Work out the finished part from the listing and answer in its coordinate system (mm). A direction names the side the tool comes from. Give positions to 0.01 mm unless a question says otherwise; leave off trailing zeros. Write each loop counter-clockwise with the first axis right and the second up, starting at its lowest first coordinate (ties: lowest second). Pieces come first, ordered by that corner, then holes.
1) Determine the mould class of faces 6 (the face through (-107, 7, 2)), 7 (the face through (9.493, 0.986, -0.36)), 8 (the face through (-2.44, 0.99, -0.54)) for opening direction X: pulls with the +X half, pulls with the -X half, needs draft (parallel to the pull), parting line crosses it, or undercut.
2) A tool of negligible diameter and unlimited length cuts with its end or side. For faces 1 (the face through (9.493, 13.986, -0.36)), 2 (the face through (-90, 15, 1)), 3 (the face through (-12.3, 4.9, -2)), 4 (the face through (-10.633, 3.595, -0.479)), 5 (the face through (-4.88, 13.99, -1.08)), from which of +Z, -Z, +X, -X, +Y, -Y can it reach the whole face along a straight path? Write none if from no direction.
3) Find section A-A (z = -6.75). Determine the outline of the cut face in (x, y), plus the area to 3 significant figures.
4) Find section B-B (x = -11.5). Determine the outline of the cut face in (y, z).
5) Find section C-C (x = -186). Determine the outline of the cut face in (y, z).
6) Given pin 1 Ø2.5 at (x, y) = (-13, 6.5) entering from -Z; pin 2 Ø5.5 at (x, y) = (-70, 9) entering from -Z; pin 3 Ø5 at (x, y) = (-191.5, 7.5) entering from +Z, each flat-ended and moving along its own axis, determine where each tip first touches the part or whether it passes through.
7) Straight lines are drawn through the part: probe 1 along Y at (x, z) = (-11.5, 2.6); probe 2 along Y at (x, z) = (-145, 1.25); probe 3 along Z at (x, y) = (-192, 0.85). For each, find the intervals that lie inside material, in ascending order.
```python
from build123d import *

# Parameters (mm, degrees)
SKETCH1_R                         = 2.5
BOSS_EXTRUDE3_DEPTH               = 2
SKETCH5_W                         = 2
SKETCH5_H                         = 11
BOSS_EXTRUDE4_DEPTH               = 197.88316
SKETCH6_R                         = 5
BOSS_EXTRUDE5_DEPTH               = 2
SKETCH8_W                         = 2
SKETCH8_H                         = 11
BOSS_EXTRUDE6_DEPTH               = 4
CUT_EXTRUDE8_REACH                = 209.363
SKETCH10_R                        = 2
SKETCH10_R_2                      = 1.5
SKETCH11_R                        = 4
SKETCH11_R_2                      = 2.5
BOSS_EXTRUDE7_DEPTH               = 4
CUT_EXTRUDE9_REACH                = 209.363
SKETCH12_R                        = 2.5
M3_5X0_6_TAPPED_HOLE2_D           = 2.9
M3_5X0_6_TAPPED_HOLE2_DEPTH       = 2
M3_5X0_6_TAPPED_HOLE2_CSINK_D     = 3.55
M3_5X0_6_TAPPED_HOLE2_CSINK_ANGLE = 90
M3_5X0_6_TAPPED_HOLE2_TIP         = 0.871247898
FILLET1_R                         = 1


with BuildPart() as part:
    # Sketch1 → Boss-Extrude3 (new body)
    with BuildSketch(Plane(origin=(0, 0, 0), x_dir=(1, 0, 0), z_dir=(0, 1, 0))):
        with BuildLine():
            Line((-206.5, 4), (-8.61684397, 4))
            ThreePointArc((-8.61684397, 4), (9.5, 0), (-8.61684397, -4))
            Line((-8.61684397, -4), (-206.5, -4))
            Line((-206.5, -4), (-206.5, 4))
        make_face()
        with Locations(Location((0, 0, 0), (0, 0, 270))):
            Circle(SKETCH1_R, mode=Mode.SUBTRACT)
    extrude(amount=BOSS_EXTRUDE3_DEPTH)

    # Sketch5 → Boss-Extrude4 (add)
    with BuildSketch(Plane.ZY.offset(206.5)):
        with Locations((3, 7.5)):
            Rectangle(SKETCH5_W, SKETCH5_H)
    extrude(amount=-BOSS_EXTRUDE4_DEPTH)


with BuildPart() as boss_extrude5_tool:
    # Sketch6 → Boss-Extrude5 (new body)
    with BuildSketch(Plane(origin=(0, 13, 0), x_dir=(1, 0, 0), z_dir=(0, 1, 0))):
        with BuildLine():
            Line((-206.5, 4), (-8.61684397, 4))
            ThreePointArc((-8.61684397, 4), (9.5, 0), (-8.61684397, -4))
            Line((-8.61684397, -4), (-206.5, -4))
            Line((-206.5, -4), (-206.5, 4))
        make_face()
        with Locations(Location((0, 0, 0), (0, 0, 270))):
            Circle(SKETCH6_R, mode=Mode.SUBTRACT)
    extrude(amount=BOSS_EXTRUDE5_DEPTH)


with BuildPart() as part_1:
    add(part.part)


with BuildPart() as part_2:
    # Boss-Extrude5: joined with boss_extrude5_tool
    add(part_1.part.fuse(boss_extrude5_tool.part, tol=0.00001))

    # Sketch8 → Boss-Extrude6 (add)
    with BuildSketch(Plane(origin=(-8.61684397, 0, 0), x_dir=(0, 0, -1), z_dir=(1, 0, 0))):
        with Locations((-3, 7.5)):
            Rectangle(SKETCH8_W, SKETCH8_H)
    extrude(amount=BOSS_EXTRUDE6_DEPTH)

    # Sketch10 → Cut-Extrude8 (cut, up to next)
    with BuildSketch(Plane(origin=(0, 0, 2), x_dir=(-1, 0, 0), z_dir=(0, 0, -1)), mode=Mode.PRIVATE) as cut_extrude8_sk1:
        with Locations((201.5, 7.5)):
            Circle(SKETCH10_R)
    cut_extrude8_tool1 = extrude(cut_extrude8_sk1.sketch, amount=-CUT_EXTRUDE8_REACH, mode=Mode.PRIVATE) & part_2.part
    # Sketch10 → Cut-Extrude8 (cut, up to next)
    with BuildSketch(Plane(origin=(0, 0, 2), x_dir=(-1, 0, 0), z_dir=(0, 0, -1)), mode=Mode.PRIVATE) as cut_extrude8_sk2:
        with Locations((191.5, 7.5)):
            Circle(SKETCH10_R)
    cut_extrude8_tool2 = extrude(cut_extrude8_sk2.sketch, amount=-CUT_EXTRUDE8_REACH, mode=Mode.PRIVATE) & part_2.part
    # Sketch10 → Cut-Extrude8 (cut, up to next)
    with BuildSketch(Plane(origin=(0, 0, 2), x_dir=(-1, 0, 0), z_dir=(0, 0, -1)), mode=Mode.PRIVATE) as cut_extrude8_sk3:
        with Locations((158.9, 7)):
            Circle(SKETCH10_R_2)
    cut_extrude8_tool3 = extrude(cut_extrude8_sk3.sketch, amount=-CUT_EXTRUDE8_REACH, mode=Mode.PRIVATE) & part_2.part
    # Sketch10 → Cut-Extrude8 (cut, up to next)
    with BuildSketch(Plane(origin=(0, 0, 2), x_dir=(-1, 0, 0), z_dir=(0, 0, -1)), mode=Mode.PRIVATE) as cut_extrude8_sk4:
        with Locations((140.9, 7)):
            Circle(SKETCH10_R_2)
    cut_extrude8_tool4 = extrude(cut_extrude8_sk4.sketch, amount=-CUT_EXTRUDE8_REACH, mode=Mode.PRIVATE) & part_2.part
    add(cut_extrude8_tool1.solids().sort_by_distance((-201.5, 7.5, 2))[0], mode=Mode.SUBTRACT)
    add(cut_extrude8_tool2.solids().sort_by_distance((-191.5, 7.5, 2))[0], mode=Mode.SUBTRACT)
    add(cut_extrude8_tool3.solids().sort_by_distance((-158.9, 7, 2))[0], mode=Mode.SUBTRACT)
    add(cut_extrude8_tool4.solids().sort_by_distance((-140.9, 7, 2))[0], mode=Mode.SUBTRACT)

    # Sketch11 → Boss-Extrude7 (add)
    with BuildSketch(Plane(origin=(0, 0, 2), x_dir=(-1, 0, 0), z_dir=(0, 0, -1))):
        with Locations((11.5, 7.5)):
            Circle(SKETCH11_R)
        with Locations((11.5, 7.5)):
            Circle(SKETCH11_R_2, mode=Mode.SUBTRACT)
    extrude(amount=BOSS_EXTRUDE7_DEPTH)

    # Sketch12 → Cut-Extrude9 (cut, up to next)
    with BuildSketch(Plane(origin=(0, 0, 2), x_dir=(-1, 0, 0), z_dir=(0, 0, -1)), mode=Mode.PRIVATE) as cut_extrude9_sk1:
        with Locations((11.5, 7.5)):
            Circle(SKETCH12_R)
    cut_extrude9_tool1 = extrude(cut_extrude9_sk1.sketch, amount=-CUT_EXTRUDE9_REACH, mode=Mode.PRIVATE) & part_2.part
    add(cut_extrude9_tool1.solids().sort_by_distance((-11.5, 7.5, 2))[0], mode=Mode.SUBTRACT)

    # M3.5x0.6 Tapped Hole2
    with Locations(Plane(origin=(0, 0, 0), x_dir=(-1, 0, 0), z_dir=(0, -1, 0))):
        with Locations((192, 0), (176, 0)):
            CounterSinkHole(M3_5X0_6_TAPPED_HOLE2_D / 2, M3_5X0_6_TAPPED_HOLE2_CSINK_D / 2, depth=M3_5X0_6_TAPPED_HOLE2_DEPTH, counter_sink_angle=M3_5X0_6_TAPPED_HOLE2_CSINK_ANGLE)
            with Locations((0, 0, -(M3_5X0_6_TAPPED_HOLE2_DEPTH + M3_5X0_6_TAPPED_HOLE2_TIP / 2))):  # 118° drill point
                Cone(0, M3_5X0_6_TAPPED_HOLE2_D / 2, M3_5X0_6_TAPPED_HOLE2_TIP, mode=Mode.SUBTRACT)

    # Fillet1
    fillet1_edges = [part_2.edges().sort_by_distance(p)[0] for p in [
        (-7.5, 7.5, 2),
    ]]
    fillet(fillet1_edges, radius=FILLET1_R)


solid = part_2.part
```
Results:
1. face 6: needs draft
1. face 7: parting line crosses it
1. face 8: undercut
2. face 1: +Y, -Y
2. face 2: +Z, -Z, +X, -X, +Y
2. face 3: -Z, +X, -X
2. face 4: -Z
2. face 5: +Y
3. outline: (-6.68, 0) - (6.68, 0) - (6.68, 2) - (-6.68, 2) - close; (-6.68, 13) - (6.68, 13) - (6.68, 15) - (-6.68, 15) - close
3. area: 53.5 mm2
4. outline: (0, -4) - (2, -4) - (2, 2) - (2.5, 2) arc R1 cw to (3.5, 1) - (3.5, -2) - (5, -2) - (5, 4) - (0, 4) - close; (10, -2) - (11.5, -2) - (11.5, 1) arc R1 cw to (12.5, 2) - (13, 2) - (13, -4) - (15, -4) - (15, 4) - (10, 4) - close
5. outline: (0, -4) - (2, -4) - (2, 2) - (13, 2) - (13, -4) - (15, -4) - (15, 4) - (0, 4) - close
6. pin 1: stops at z = -2
6. pin 2: stops at z = 2
6. pin 3: stops at z = 4
7. probe 1: y = 0 to 5, 10 to 15
7. probe 2: y = 0 to 2, 13 to 15
7. probe 3: z = -4 to -1.45, 1.45 to 4
